Build history of the part. All positions in model axes, mm. A direction names the side the tool comes from. Give positions to 0.01 mm unless a question says otherwise; leave off trailing zeros. Write each loop counter-clockwise with the first axis right and the second up, starting at its lowest first coordinate (ties: lowest second). Pieces come first, ordered by that corner, then holes. Notation, with made-up numbers: M 33.25,58.5 L 67.25,58.5 A29 ccw 67.25,80.5 Z; hole C 72,56 d5. An arc over 180 degrees is marked long. Return JSON: item names as keys, results as strings. Group by question number.
Q1. Flat gauge pins, fed straight in: pin 1 Ø10 at (x, y) = (5, -3.5) entering from -Z; pin 2 Ø10 at (x, y) = (8, 4) entering from +Z; pin 3 Ø1.8 at (y, z) = (1, -4) entering from +X. Where does each tip first touch, or does it go through?
Q2. Pull direction Z, two halves, no side cores. Call faces 1 (the flat face through (-2.1, 10, 0.2)), 2 (the flat face through (-30, 0, 3)), 3 (the flat face through (-13, 2, -3)), 4 (the flat face through (10, 0, 0)): +Z half, -Z half, draft (parallel to the pull), parting line (faces both ways), or undercut.
Q3. Band-saw the part on A-A, the plane x = -21.75. Give the cut face in (y, z).
Q4. Band-saw the part on B-B, the plane z = -1.5. Give the cut face in (x, y).
Q5. Wall check: probe 1 along X at (y, z) = (2, 10); probe 2 along X at (y, z) = (6.75, -2.75); probe 3 along X at (y, z) = (-3, 7.75). Give the ranges that are in metal, low to high.
Q6. Band-saw the part on D-D, the plane x = 0.5. Give the cut face in (y, z).
Q7. Tool access for faces 5 (the flat face through (-22, 0, -6)), 6 (the flat face through (-27.75, 0, 7)), 7 (the cylindrical face through (-15.886, 0.14, 11.27)), 8 (the cylindrical face through (21.86, -0.14, 6)): list every direction of +Z, -Z, +X, -X, +Y, -Y with a clear straight run to the whole face (end or side of a thin tool).
from build123d import *

# Parameters (mm, degrees)
F0_W      = 54.5
F0_H      = 20
F1_DEPTH  = 3
F3_DEPTH  = 10
F4_R      = 2
F5_R      = 0.5
F7_DEPTH  = 10
F9_DEPTH  = 20
F10_W     = 6
F10_H     = 6
F11_DEPTH = 8


with BuildPart() as f1:
    # F0 (on Top) → F1 (new body)
    with BuildSketch(Plane.XY):
        Rectangle(F0_W, F0_H)
    extrude(amount=F1_DEPTH)

    # F2 (on Front) → F3 (join, symmetric)
    with BuildSketch(Plane.XZ):
        with BuildLine():
            Line((-15.75, 0), (-15.75, 10))
            ThreePointArc((-15.75, 10), (-15.9544450423, 11.5529142706), (-16.5538475773, 13))
            Line((-16.5538475773, 13), (-18.2858983849, 12))
            ThreePointArc((-18.2858983849, 12), (-21.75, 6), (-25.2141016151, 12))
            Line((-25.2141016151, 12), (-26.9461524227, 13))
            ThreePointArc((-26.9461524227, 13), (-27.5455549577, 11.5529142706), (-27.75, 10))
            Line((-27.75, 10), (-27.75, 0))
            Line((-27.75, 0), (-15.75, 0))
        make_face()
        with BuildLine():
            ThreePointArc((25.2141016151, 12), (21.75, 6), (18.2858983849, 12))
            Line((18.2858983849, 12), (16.5538475773, 13))
            ThreePointArc((16.5538475773, 13), (15.9544450423, 11.5529142706), (15.75, 10))
            Line((15.75, 10), (15.75, 0))
            Line((15.75, 0), (27.75, 0))
            Line((27.75, 0), (27.75, 10))
            ThreePointArc((27.75, 10), (27.5455549577, 11.5529142706), (26.9461524227, 13))
            Line((26.9461524227, 13), (25.2141016151, 12))
        make_face()
    extrude(amount=F3_DEPTH, both=True)

    # F4
    f4_edges = [f1.edges().sort_by_distance(p)[0] for p in [
        (-15.75, 0, 3),
        (15.75, 0, 3),
    ]]
    fillet(f4_edges, radius=F4_R)

    # F5
    f5_edges = [f1.edges().sort_by_distance(p)[0] for p in [
        (-26.946152, 0, 13),
        (-25.214102, 0, 12),
        (-18.285898, 0, 12),
        (-16.553848, 0, 13),
        (18.285898, 0, 12),
        (16.553848, 0, 13),
        (25.214102, 0, 12),
        (26.946152, 0, 13),
    ]]
    fillet(f5_edges, radius=F5_R)

    # F6 (on Front) → F7 (join, symmetric)
    with BuildSketch(Plane.XZ):
        Polygon((-7.75, -8), (-7.75, 0), (-10.25, 0), (-10.25, -6), (-30.25, -6), (-30.25, 0), (-32.75, 0), (-32.75, -8), align=None)
    extrude(amount=F7_DEPTH, both=True)

    # F8 (on face) → F9 (join)
    with BuildSketch(Plane.XZ.offset(10)):
        Polygon((-30.25, 0), (-27.75, 0), (-27.75, 3), (-32.75, 3), (-32.75, 0), align=None)
    extrude(amount=-F9_DEPTH)

    # F10 (on face) → F11 (join)
    with BuildSketch(Plane(origin=(0, 10, 0), x_dir=(-1, 0, 0), z_dir=(0, 1, 0))):
        with Locations((13.25, -3)):
            Rectangle(F10_W, F10_H)
    extrude(amount=-F11_DEPTH)


solid = f1.part
From the geometry:
{
 "1": {"pin 1": "stops at z = 0", "pin 2": "stops at z = 3", "pin 3": "stops at x = -7.75"},
 "2": {"face 1": "draft", "face 2": "+Z half", "face 3": "undercut", "face 4": "-Z half"},
 "3": {"outline": "M -10,-8 L 10,-8 L 10,-6 L -10,-6 Z; M -10,0 L 10,0 L 10,6 L -10,6 Z"},
 "4": {"outline": "M -32.75,-10 L -30.25,-10 L -30.25,10 L -32.75,10 Z; M -16.25,2 L -10.25,2 L -10.25,-10 L -7.75,-10 L -7.75,10 L -16.25,10 Z"},
 "5": {"probe 1": "x = -27.75 to -25.75, -17.75 to -15.75, 15.75 to 17.75, 25.75 to 27.75", "probe 2": "x = -32.75 to -30.25, -16.25 to -7.75", "probe 3": "x = -27.75 to -25.06, -18.44 to -15.75, 15.75 to 18.44, 25.06 to 27.75"},
 "6": {"outline": "M -10,0 L 10,0 L 10,3 L -10,3 Z"},
 "7": {"face 5": "-Y", "face 6": "+Z, -X, +Y, -Y", "face 7": "+Z, +Y, -Y", "face 8": "+Y, -Y"}
}
